For this review, take the finished solid that the model builds, in its own axes (mm). A direction names the side the tool comes from. Coordinates: 2 decimals unless noted, no trailing zeros. Loops run counter-clockwise (first coordinate to the right, second up) from the corner with the lowest first, then second, coordinate; pieces in that order, holes last. Notation, with made-up numbers: M 7.5,48.25 L 15.5,48.25 A31 cw 15.5,77.25 Z; hole C 25,-13.75 d9. An arc over 180 degrees is marked long. Write item = value, one per line.
Autodesk Inventor part; units mm, degrees
ref_plane "YZ Plane" through (0, 0, 0) normal (1, 0, 0) x (0, 1, 0)
ref_plane "XZ Plane" through (0, 0, 0) normal (0, 1, 0) x (-1, 0, 0)
ref_plane "XY Plane" through (0, 0, 0) normal (0, 0, 1) x (1, 0, 0)
sketch "Skizze1" plane through (0, 0, 0) normal (0, 0, 1) x (1, 0, 0)
  circle A0 centre (-11.2583, 6.5) radius 1.5
  circle A1 centre (-11.2583, -6.5) radius 1.5
  circle A2 centre (0, -13) radius 1.5
  circle A3 centre (11.2583, -6.5) radius 1.5
  circle A4 centre (11.2583, 6.5) radius 1.5
  circle A5 centre (0, 13) radius 1.5
  arc A6 (14.3761, 1.8914) -> (11.9393, 3.5783) centre (12.3932, 1.6305) ccw
  arc A7 (14.3761, -1.8914) -> (14.3761, 1.8914) centre (0, 0) ccw
  arc A8 (11.9393, -3.5783) -> (14.3761, -1.8914) centre (12.3932, -1.6305) ccw
  arc A9 (11.9393, -3.5783) -> (9.0685, -8.5505) centre (11.2583, -6.5) ccw
  arc A10 (8.826, -11.5044) -> (9.0685, -8.5505) centre (7.6087, -9.9176) ccw
  arc A11 (5.5501, -13.3958) -> (8.826, -11.5044) centre (0, 0) ccw
  arc A12 (2.8707, -12.1288) -> (5.5501, -13.3958) centre (4.7846, -11.5481) ccw
  arc A13 (2.8707, -12.1288) -> (-2.8707, -12.1288) centre (0, -13) ccw
  arc A14 (-5.5501, -13.3958) -> (-2.8707, -12.1288) centre (-4.7846, -11.5481) ccw
  arc A15 (-8.826, -11.5044) -> (-5.5501, -13.3958) centre (0, 0) ccw
  arc A16 (-9.0685, -8.5505) -> (-8.826, -11.5044) centre (-7.6087, -9.9176) ccw
  arc A17 (-9.0685, -8.5505) -> (-11.9393, -3.5783) centre (-11.2583, -6.5) ccw
  arc A18 (-14.3761, -1.8914) -> (-11.9393, -3.5783) centre (-12.3932, -1.6305) ccw
  arc A19 (-14.3761, 1.8914) -> (-14.3761, -1.8914) centre (0, 0) ccw
  arc A20 (-11.9393, 3.5783) -> (-14.3761, 1.8914) centre (-12.3932, 1.6305) ccw
  arc A21 (-11.9393, 3.5783) -> (-9.0685, 8.5505) centre (-11.2583, 6.5) ccw
  arc A22 (-8.826, 11.5044) -> (-9.0685, 8.5505) centre (-7.6087, 9.9176) ccw
  arc A23 (-5.5501, 13.3958) -> (-8.826, 11.5044) centre (0, 0) ccw
  arc A24 (-2.8707, 12.1288) -> (-5.5501, 13.3958) centre (-4.7846, 11.5481) ccw
  arc A25 (-2.8707, 12.1288) -> (2.8707, 12.1288) centre (0, 13) ccw
  arc A26 (5.5501, 13.3958) -> (2.8707, 12.1288) centre (4.7846, 11.5481) ccw
  arc A27 (8.826, 11.5044) -> (5.5501, 13.3958) centre (0, 0) ccw
  arc A28 (9.0685, 8.5505) -> (8.826, 11.5044) centre (7.6087, 9.9176) ccw
  arc A29 (9.0685, 8.5505) -> (11.9393, 3.5783) centre (11.2583, 6.5) ccw
  circle A30 centre (0, 0) radius 17.5
  circle A31 centre (0, 0) radius 19.5
  point P0 (0, 0)
  dimension "d0" = 39
extrude "Extrusion1" add sketch "Skizze1" along normal blind 5 contours A7 A8 A9 A10 A11 A12 A13 A14 A15 A16 A17 A18 A19 A20 A21 A22 A23 A24 A25 A26 A27 A28 A29 A6 | A30 | A31
sketch "Skizze2" plane through (0, 0, 5) normal (0, 0, 1) x (1, 0, 0)
  circle A0 centre (0, 0) radius 7.5
  dimension "d3" = 15
extrude "Extrusion2" add sketch "Skizze2" along normal blind 5
sketch "Skizze6" plane through (0, 0, 5) normal (0, 0, 1) x (1, 0, 0)
  circle A0 centre (0, 0) radius 7.5
  circle A1 centre (0, 13) radius 1.5
  circle A2 centre (11.2583, 6.5) radius 1.5
  circle A3 centre (11.2583, -6.5) radius 1.5
  circle A4 centre (0, -13) radius 1.5
  circle A5 centre (-11.2583, -6.5) radius 1.5
  circle A6 centre (-11.2583, 6.5) radius 1.5
  circle A7 centre (0, 0) radius 19.5
  circle A8 centre (11.2583, 6.5) radius 3.5
  dimension "d20" = 7
fillet "Rundung1" radius 5 1 edges at (-7.5, 0, 5)
fillet "Rundung2" radius 2 1 edges at (-7.5, 0, 10)
sketch "Skizze3" plane through (0, 0, 0) normal (0, 0, -1) x (-1, 0, 0)
  line L0 (0, -4.0415) -> (-3.5, -2.0207)
  line L1 (-3.5, -2.0207) -> (-3.5, 2.0207)
  line L2 (-3.5, 2.0207) -> (0, 4.0415)
  line L3 (0, 4.0415) -> (3.5, 2.0207)
  line L4 (3.5, 2.0207) -> (3.5, -2.0207)
  line L5 (3.5, -2.0207) -> (0, -4.0415)
  point P0 (0, 0)
  point P1 (0, 0)
  dimension "d8" = 7
sketch "Skizze4" plane through (0, 0, 10) normal (0, 0, 1) x (1, 0, 0)
  point P0 (0, 0)
hole "Bohrung1" at (0, 0, 10) direction (0, 0, -1) diameter 4 end through all
extrude "Extrusion3" cut sketch "Skizze3" against normal blind 3
sketch "Skizze5" plane through (0, 0, 3) normal (0, 0, -1) x (-1, 0, 0)
  circle A0 centre (0, 0) radius 2
  circle A1 centre (0, 0) radius 2
extrude "Extrusion4" add sketch "Skizze5" against normal blind 0.2
extrude "Extrusion5" cut sketch "Skizze6" along normal blind 10 contours A2 | A8
pattern_circular "Runde Anordnung1" count 6 over 360 about axis through (0, 0, -46.0535) along (0, 0, 1) of "Extrusion5"
properties part number "GripperMountPlatehock" material "ABS-Kunststoff"
Q1. Machinability: for faces 1 (the face through (-9, 5, 5)), 2 (the face through (0, 0, 3)), 3 (the face through (0.1, 9.5, 5.4)), 4 (the face through (-9.87, 7.07, 2.46)), which of the approach directions +Z, -Z, +X, -X, +Y, -Y give a long, thin tool a straight path to every point of the face, cutting with its end or side? Answer none if there is none.
Solved:
face_1 = +Z
face_2 = -Z
face_3 = +Z, +Y
face_4 = +Z, -Z
Q2. Add section D-D (y = 6.5). State how many separate pieces and enclosed holes the cut face has, and give its area (3 significant figures).
Solved:
separate_pieces = 3
enclosed_holes = 0
area = 205 mm²
Q3. For line 1 along Y through (x, z) = (0, 3.1); line 2 along X through (y, z) = (-0.5, 0.75); line 3 along Y through (x, z) = (-0.5, 3.75), list the stretches that pass through material, from the lowest coordinate up.
Solved:
line_1 = -19.5 to -14.5, -11.5 to 11.5, 14.5 to 19.5
line_2 = -19.49 to -3.5, 3.5 to 19.49
line_3 = -19.49 to -14.41, -11.59 to -1.94, 1.94 to 11.59, 14.41 to 19.49
Q4. For pin 1 Ø4 at (x, y) = (0, 13) entering from -Z; pin 2 Ø1 at (x, z) = (-6, 8) entering from +Y; pin 3 Ø2.5 at (x, y) = (0, 0) entering from -Z; pin 4 Ø5 at (x, y) = (-11.26, -6.5) entering from +Z, all flat-tipped, find the tip position at first contact; note any pin that passes through.
Solved:
pin_1 = 0
pin_2 = 5.8
pin_3 = 3
pin_4 = 5
Q5. Add section B-B (z = 2.5). Write out the cut boundary in (x, y), and give its area (3 significant figures).
Solved:
outline = C 0,0 d39; hole C -11.26,-6.5 d3; hole C -11.26,6.5 d3; hole M -3.5,-2.02 L 0,-4.04 L 3.5,-2.02 L 3.5,2.02 L 0,4.04 L -3.5,2.02 Z; hole C 0,-13 d3; hole C 0,13 d3; hole C 11.26,-6.5 d3; hole C 11.26,6.5 d3
area = 1,110 mm²
Q6. Add section C-C (z = 4.5). Write out the cut boundary in (x, y), and give its area (3 significant figures).
Solved:
outline = C 0,0 d39; hole C -11.26,-6.5 d3; hole C -11.26,6.5 d3; hole C 0,0 d4; hole C 0,-13 d3; hole C 0,13 d3; hole C 11.26,-6.5 d3; hole C 11.26,6.5 d3
area = 1,140 mm²
Q7. Draft analysis for pull direction Y (two halves, no side actions). For faces 5 (the face through (-1.726, 3.045, 1.479)), 6 (the face through (-0.1, -9.5, 5.4)), 7 (the face through (-1, 2, 10)), state which applies: +Y half, -Y half, draft (parallel to the pull), parting line (faces both ways), or undercut.
Solved:
face_5 = undercut
face_6 = -Y half
face_7 = draft
Q8. Add section A-A (y = -14). Write out the cut boundary in (x, z), and give its area (3 significant figures).
Solved:
outline = M -13.57,0 L -1.12,0 L -1.12,5 L -13.57,5 Z; M 1.12,0 L 13.57,0 L 13.57,5 L 1.12,5 Z
area = 125 mm²
